Here's how the part is built. I have some questions about the finished solid (model axes, mm). Coordinates: 2 decimals unless noted, no trailing zeros. Loops run counter-clockwise (first coordinate to the right, second up) from the corner with the lowest first, then second, coordinate; pieces in that order, holes last. Notation, with made-up numbers: (-2, 38) -> (8, 38) arc R8 cw to (8, 47) -> close; hole circle Ø11 at (38.5, -26.5). An arc over 180 degrees is marked (long way). Answer as a JSON object with one key per item and string values. Group by question number.
Q1. I'm going to push flat-ended pins straight in: pin 1 (2 mm diameter, centred on x = -16.51, y = -20.828, fed in from -Z); pin 2 (3 mm diameter, centred on x = 19.5, y = 1, fed in from -Z). Where does each tip first touch, or does it pass through?
Q2. Thinking about a two-plate mould opening in X: for faces 1 (the cylindrical face through (-24.676, -30.986, 1.61)), 2 (the cylindrical face through (-16.725, 26.527, 1.61)), 3 (the flat face through (25.4, 0, 2)), which applies, released by +X, released by -X, zero draft, split by the parting line, or undercut?
Q3. I want a section at A-A on y = 12.7. Write out the boundary of the cut face in (x, z) (3 decimals).
Q4. I want a section at B-B on z = 2.4. Write out the boundary of the cut face in (x, y).
Q5. I need wall thicknesses on line 1 (Y direction, x = 16.51, z = 1.55); line 2 (X direction, y = -19.5, z = 0.95); line 3 (X direction, y = 24, z = 2.9). Which ranges of each line are inside material? Lowest first, please.
```python
from build123d import *

# Parameters (mm, degrees)
SKETCH1_W                        = 50.8
SKETCH1_H                        = 63.5
BOSS_EXTRUDE1_DEPTH              = 3.175
F_10_0_1935_DIAMETER_HOLE1_D     = 4.8133
F_10_0_1935_DIAMETER_HOLE1_DEPTH = 3.175
M3_CLEARANCE_HOLE1_D             = 3.2984
M3_CLEARANCE_HOLE1_DEPTH         = 3.175
FILLET1_R                        = 2.54


with BuildPart() as part:
    # Sketch1 → Boss-Extrude1 (new body)
    with BuildSketch(Plane.XY):
        Rectangle(SKETCH1_W, SKETCH1_H)
    extrude(amount=BOSS_EXTRUDE1_DEPTH)

    # #10 (0.1935) Diameter Hole1
    with Locations(Plane(origin=(0, 0, 0), x_dir=(-1, 0, 0), z_dir=(0, 0, -1))):
        with Locations((-18.542, 12.7), (18.542, 12.7)):
            Hole(F_10_0_1935_DIAMETER_HOLE1_D / 2, depth=F_10_0_1935_DIAMETER_HOLE1_DEPTH)

    # M3 Clearance Hole1
    with Locations(Plane(origin=(0, 0, 0), x_dir=(-1, 0, 0), z_dir=(0, 0, -1))):
        with Locations((-16.51, 24.892), (16.51, 24.892), (-16.51, -20.828), (16.51, -20.828)):
            Hole(M3_CLEARANCE_HOLE1_D / 2, depth=M3_CLEARANCE_HOLE1_DEPTH)

    # Fillet1
    fillet1_edges = [part.edges().sort_by_distance(p)[0] for p in [
        (25.4, -31.75, 1.5875),
        (-25.4, -31.75, 1.5875),
        (-25.4, 31.75, 1.5875),
        (25.4, 31.75, 1.5875),
    ]]
    fillet(fillet1_edges, radius=FILLET1_R)


solid = part.part
```
Result set:
{
 "1": {"pin 1": "passes through", "pin 2": "stops at z = 0"},
 "2": {"face 1": "released by -X", "face 2": "undercut", "face 3": "released by +X"},
 "3": {"outline": "(-25.4, 0) -> (-20.949, 0) -> (-20.949, 3.175) -> (-25.4, 3.175) -> close; (-16.135, 0) -> (16.135, 0) -> (16.135, 3.175) -> (-16.135, 3.175) -> close; (20.949, 0) -> (25.4, 0) -> (25.4, 3.175) -> (20.949, 3.175) -> close"},
 "4": {"outline": "(-25.4, -29.21) arc R2.54 ccw to (-22.86, -31.75) -> (22.86, -31.75) arc R2.54 ccw to (25.4, -29.21) -> (25.4, 29.21) arc R2.54 ccw to (22.86, 31.75) -> (-22.86, 31.75) arc R2.54 ccw to (-25.4, 29.21) -> close; hole circle Ø4.81 at (-18.54, 12.7); hole circle Ø3.3 at (-16.51, -20.83); hole circle Ø3.3 at (-16.51, 24.89); hole circle Ø3.3 at (16.51, -20.83); hole circle Ø3.3 at (16.51, 24.89); hole circle Ø4.81 at (18.54, 12.7)"},
 "5": {"line 1": "y = -31.75 to -22.48, -19.18 to 11.41, 13.99 to 23.24, 26.54 to 31.75", "line 2": "x = -25.4 to -17.49, -15.53 to 15.53, 17.49 to 25.4", "line 3": "x = -25.4 to -17.9, -15.12 to 15.12, 17.9 to 25.4"}
}
